Here's how the part is built. I have some questions about the finished solid (model axes, mm). A direction names the side the tool comes from. Round coordinates to 2 decimals unless told otherwise and drop trailing zeros. Loops run counter-clockwise (first coordinate to the right, second up) from the corner with the lowest first, then second, coordinate; pieces in that order, holes last. Notation, with made-up numbers: (5, 59.25) -> (19, 59.25) arc R8 ccw to (19, 65.25) -> close; hole circle Ø5 at (87, 10.5). An arc over 180 degrees is marked (long way). Use one line per item in the form item = value. Start each with the question number.
Item 1: I'm going to push flat-ended pins straight in: pin 1 Ø7 at (x, z) = (24, -19) entering from +Y; pin 2 Ø10 at (x, z) = (39, -196) entering from +Y; pin 3 Ø5 at (x, z) = (133, -30) entering from -Y (3 decimals); pin 4 Ø10 at (y, z) = (32, -128) entering from +X. Where does each tip first touch, or does it pass through?
Item 2: If we section it at B-B (y = 28.5): Write out the boundary of the cut face in (x, z).
Item 3: If we section it at A-A (z = -105): Write out the boundary of the cut face in (x, y).
Item 4: If I drill on L1, parallel to X at y = 50.3, z = -17.5; L2, parallel to X at y = 85.5, z = -6; L3, parallel to Z at x = 98, y = 50.4, over which ranges is the centre line in solid material (lowest first)? Write a range as [from, to].
Item 5: If we section it at C-C (z = -144.5): Write out the boundary of the cut face in (x, y), then the cut area to 3 significant figures.
Item 6: If we section it at D-D (y = 85): State how many separate pieces and enclosed holes the cut face has, then the cut area to 3 significant figures.
Item 7: For faces 1 (the face through (8, 81, -9)), 2 (the face through (132, 4, -60)), 3 (the face through (111, 82, -214)), 4 (the face through (8, 86, -208)), which set-ups out of +Z, -Z, +X, -X, +Y, -Y let a thin tool reach every point of the face, with its end or its side?
Item 8: Thinking about a two-plate mould opening in Y: for faces 5 (the face through (111, 86, -8)), 6 (the face through (61, 91, -3)), 7 (the face through (119, 37, -106)), which applies, released by +Y, released by -Y, zero draft, split by the parting line, or undercut?
```python
from build123d import *

# Parameters (mm, degrees)
SKETCH1_W           = 123
SKETCH1_H           = 220
BOSS_EXTRUDE1_DEPTH = 4
SKETCH2_W           = 123
SKETCH2_H           = 220
SKETCH2_W_2         = 115
SKETCH2_H_2         = 212
BOSS_EXTRUDE2_DEPTH = 87
CUT_EXTRUDE1_REACH  = 269.974
SKETCH3_W           = 115
SKETCH3_H           = 45
SKETCH4_W           = 150
SKETCH4_H           = 30
CUT_EXTRUDE2_DEPTH  = 268.973879324
SKETCH6_W           = 24
SKETCH6_H           = 37
SKETCH6_R           = 1.45
BOSS_EXTRUDE4_DEPTH = 3
SKETCH8_W           = 12
SKETCH8_H           = 12
BOSS_EXTRUDE5_DEPTH = 10
CUT_EXTRUDE3_REACH  = 269.974
SKETCH9_R           = 1.95
CUT_EXTRUDE4_REACH  = 269.974
SKETCH10_W          = 99
SKETCH10_H          = 35
CHAMFER1_SIZE       = 10
SKETCH11_W          = 20
SKETCH11_H          = 120
SKETCH11_R          = 3
BOSS_EXTRUDE6_DEPTH = 4
CHAMFER3_SIZE       = 2
CHAMFER4_SIZE       = 3


with BuildPart() as part:
    # Sketch1 → Boss-Extrude1 (new body)
    with BuildSketch(Plane(origin=(0, 0, 0), x_dir=(1, 0, 0), z_dir=(0, 1, 0))):
        with Locations((61.5, 110)):
            Rectangle(SKETCH1_W, SKETCH1_H)
    extrude(amount=BOSS_EXTRUDE1_DEPTH)

    # Sketch2 → Boss-Extrude2 (add)
    with BuildSketch(Plane(origin=(0, 4, 0), x_dir=(1, 0, 0), z_dir=(0, 1, 0))):
        with Locations((61.5, 110)):
            Rectangle(SKETCH2_W, SKETCH2_H)
        with Locations((61.5, 110)):
            Rectangle(SKETCH2_W_2, SKETCH2_H_2, mode=Mode.SUBTRACT)
    extrude(amount=BOSS_EXTRUDE2_DEPTH)

    # Sketch3 → Cut-Extrude1 (cut, up to next)
    with BuildSketch(Plane.XY, mode=Mode.PRIVATE) as cut_extrude1_sk1:
        with Locations((61.5, 26.5)):
            Rectangle(SKETCH3_W, SKETCH3_H)
    cut_extrude1_tool1 = extrude(cut_extrude1_sk1.sketch, amount=-CUT_EXTRUDE1_REACH, mode=Mode.PRIVATE) & part.part
    add(cut_extrude1_tool1.solids().sort_by_distance((61.5, 26.5, 0))[0], mode=Mode.SUBTRACT)

    # Sketch4 → Cut-Extrude2 (cut, through all)
    with BuildSketch(Plane(origin=(123, 0, 0), x_dir=(0, 0, -1), z_dir=(1, 0, 0))):
        with Locations((125, 76)):
            Rectangle(SKETCH4_W, SKETCH4_H)
    extrude(amount=-CUT_EXTRUDE2_DEPTH, mode=Mode.SUBTRACT)

    # Sketch6 → Boss-Extrude4 (add)
    # profile 1 of 2: a face of its own
    with BuildSketch(Plane(origin=(0, 49, 0), x_dir=(-1, 0, 0), z_dir=(0, -1, 0))):
        with Locations((-16, 22.5)):
            Rectangle(SKETCH6_W, SKETCH6_H)
        with Locations(Location((-25, 27.5, 0), (0, 0, 90))):
            Circle(SKETCH6_R, mode=Mode.SUBTRACT)
        with Locations(Location((-25, 17.5, 0), (0, 0, 270))):
            Circle(SKETCH6_R, mode=Mode.SUBTRACT)
    # profile 2 of 2: a face of its own
    with BuildSketch(Plane(origin=(0, 49, 0), x_dir=(-1, 0, 0), z_dir=(0, -1, 0))):
        with Locations((-107, 22.5)):
            Rectangle(SKETCH6_W, SKETCH6_H)
        with Locations(Location((-98, 17.5, 0), (0, 0, 90))):
            Circle(SKETCH6_R, mode=Mode.SUBTRACT)
        with Locations(Location((-98, 27.5, 0), (0, 0, 270))):
            Circle(SKETCH6_R, mode=Mode.SUBTRACT)
    extrude(amount=-BOSS_EXTRUDE4_DEPTH)

    # Sketch8 → Boss-Extrude5 (add)
    with BuildSketch(Plane(origin=(0, 91, 0), x_dir=(1, 0, 0), z_dir=(0, 1, 0))):
        with Locations((117, 214)):
            Rectangle(SKETCH8_W, SKETCH8_H)
        with Locations((6, 214)):
            Rectangle(SKETCH8_W, SKETCH8_H)
        with Locations((117, 6)):
            Rectangle(SKETCH8_W, SKETCH8_H)
        with Locations((6, 6)):
            Rectangle(SKETCH8_W, SKETCH8_H)
    extrude(amount=-BOSS_EXTRUDE5_DEPTH)

    # Sketch9 → Cut-Extrude3 (cut, up to next)
    with BuildSketch(Plane(origin=(0, 91, 0), x_dir=(1, 0, 0), z_dir=(0, 1, 0)), mode=Mode.PRIVATE) as cut_extrude3_sk1:
        with Locations(Location((6, 214, 0), (0, 0, 270))):
            Circle(SKETCH9_R)
    cut_extrude3_tool1 = extrude(cut_extrude3_sk1.sketch, amount=-CUT_EXTRUDE3_REACH, mode=Mode.PRIVATE) & part.part
    # Sketch9 → Cut-Extrude3 (cut, up to next)
    with BuildSketch(Plane(origin=(0, 91, 0), x_dir=(1, 0, 0), z_dir=(0, 1, 0)), mode=Mode.PRIVATE) as cut_extrude3_sk2:
        with Locations(Location((117, 214, 0), (0, 0, 90))):
            Circle(SKETCH9_R)
    cut_extrude3_tool2 = extrude(cut_extrude3_sk2.sketch, amount=-CUT_EXTRUDE3_REACH, mode=Mode.PRIVATE) & part.part
    # Sketch9 → Cut-Extrude3 (cut, up to next)
    with BuildSketch(Plane(origin=(0, 91, 0), x_dir=(1, 0, 0), z_dir=(0, 1, 0)), mode=Mode.PRIVATE) as cut_extrude3_sk3:
        with Locations(Location((117, 6, 0), (0, 0, 270))):
            Circle(SKETCH9_R)
    cut_extrude3_tool3 = extrude(cut_extrude3_sk3.sketch, amount=-CUT_EXTRUDE3_REACH, mode=Mode.PRIVATE) & part.part
    # Sketch9 → Cut-Extrude3 (cut, up to next)
    with BuildSketch(Plane(origin=(0, 91, 0), x_dir=(1, 0, 0), z_dir=(0, 1, 0)), mode=Mode.PRIVATE) as cut_extrude3_sk4:
        with Locations(Location((6, 6, 0), (0, 0, 90))):
            Circle(SKETCH9_R)
    cut_extrude3_tool4 = extrude(cut_extrude3_sk4.sketch, amount=-CUT_EXTRUDE3_REACH, mode=Mode.PRIVATE) & part.part
    add(cut_extrude3_tool1.solids().sort_by_distance((6, 91, -214))[0], mode=Mode.SUBTRACT)
    add(cut_extrude3_tool2.solids().sort_by_distance((117, 91, -214))[0], mode=Mode.SUBTRACT)
    add(cut_extrude3_tool3.solids().sort_by_distance((117, 91, -6))[0], mode=Mode.SUBTRACT)
    add(cut_extrude3_tool4.solids().sort_by_distance((6, 91, -6))[0], mode=Mode.SUBTRACT)

    # Sketch10 → Cut-Extrude4 (cut, up to next)
    with BuildSketch(Plane(origin=(0, 0, -220), x_dir=(-1, 0, 0), z_dir=(0, 0, -1)), mode=Mode.PRIVATE) as cut_extrude4_sk1:
        with Locations((-61.5, 73.5)):
            Rectangle(SKETCH10_W, SKETCH10_H)
    cut_extrude4_tool1 = extrude(cut_extrude4_sk1.sketch, amount=-CUT_EXTRUDE4_REACH, mode=Mode.PRIVATE) & part.part
    add(cut_extrude4_tool1.solids().sort_by_distance((61.5, 73.5, -220))[0], mode=Mode.SUBTRACT)

    # Chamfer1
    chamfer1_edges = [part.edges().sort_by_distance(p)[0] for p in [
        (119, 52, -22.5),
        (4, 52, -22.5),
    ]]
    chamfer(chamfer1_edges, length=CHAMFER1_SIZE)

    # Sketch11 → Boss-Extrude6 (add)
    with BuildSketch(Plane.XZ):
        with Locations((133, -60)):
            Rectangle(SKETCH11_W, SKETCH11_H)
        with Locations(Location((133, -105, 0), (0, 0, 270))):
            Circle(SKETCH11_R, mode=Mode.SUBTRACT)
        with Locations(Location((133, -30, 0), (0, 0, 270))):
            Circle(SKETCH11_R, mode=Mode.SUBTRACT)
    extrude(amount=-BOSS_EXTRUDE6_DEPTH)

    # Chamfer3
    chamfer3_edges = [part.edges().sort_by_distance(p)[0] for p in [
        (111, 73.5, -220),
        (61.5, 56, -220),
        (12, 73.5, -220),
        (133, 4, 0),
        (143, 4, -60),
        (123, 76, -50),
        (123, 61, -125),
        (123, 76, -200),
        (0, 45.5, -220),
        (123, 45.5, -220),
        (123, 47.5, 0),
        (0, 45.5, 0),
    ]]
    chamfer(chamfer3_edges, length=CHAMFER3_SIZE)

    # Chamfer4
    chamfer4_edges = [part.edges().sort_by_distance(p)[0] for p in [
        (133, 4, -102),
        (133, 4, -27),
    ]]
    chamfer(chamfer4_edges, length=CHAMFER4_SIZE)


solid = part.part
```
Values found:
q1.pin_1 = 52
q1.pin_2 = 4
q1.pin_3 = through
q1.pin_4 = 123
q2.outline = (0, -218) -> (2, -220) -> (121, -220) -> (123, -218) -> (123, -2) -> (121, 0) -> (119, 0) -> (119, -216) -> (4, -216) -> (4, 0) -> (2, 0) -> (0, -2) -> close
q3.outline = (0, 0) -> (130, 0) -> (130, 1) -> (127, 4) -> (123, 4) -> (123, 59) -> (121, 61) -> (119, 61) -> (119, 4) -> (4, 4) -> (4, 61) -> (0, 61) -> close; (136, 0) -> (143, 0) -> (143, 2) -> (141, 4) -> (139, 4) -> (136, 1) -> close
q4.L1 = [0, 23.55], [26.45, 28], [95, 96.55], [99.45, 123]
q4.L2 = [0, 4.05], [7.95, 12], [111, 115.05], [118.95, 123]
q4.L3 = [-220, -216], [-41, -28.95], [-26.05, -18.95], [-16.05, 0]
q5.outline = (0, 0) -> (123, 0) -> (123, 59) -> (121, 61) -> (119, 61) -> (119, 4) -> (4, 4) -> (4, 61) -> (0, 61) -> close
q5.area = 946 mm2
q6.separate_pieces = 3
q6.enclosed_holes = 4
q6.area = 1,280 mm2
q7.face_1 = none
q7.face_2 = +Z, -Z, +X, +Y
q7.face_3 = -Z, +Y
q7.face_4 = +Y
q8.face_5 = zero draft
q8.face_6 = released by +Y
q8.face_7 = undercut
